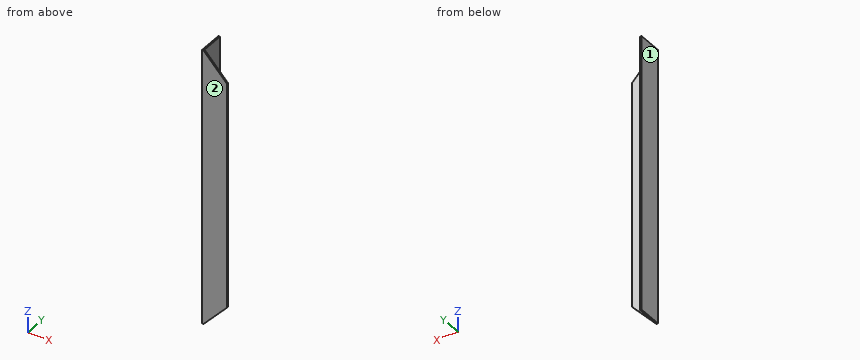
```python
from build123d import *

# Parameters (mm, degrees)
F1_DEPTH      = 533.4
F1_DEPTH_BACK = 25.4
F3_DEPTH      = 3.176


with BuildPart() as f1:
    # F0 (on Top) → F1 (new body, two sides)
    with BuildSketch(Plane.XY) as f1_sk:
        Polygon((0, 50.8), (-3.175, 50.8), (-3.175, 0), (47.625, 0), (47.625, 3.175), (0, 3.175), align=None)
    extrude(amount=F1_DEPTH)
    extrude(f1_sk.sketch, amount=-F1_DEPTH_BACK)

    # F2 (on face) → F3 (cut, through all)
    with BuildSketch(Plane(origin=(0, 3.175, 0), x_dir=(-1, 0, 0), z_dir=(0, 1, 0))):
        Polygon((-47.625, 533.4), (-47.625, 482.6), (0, 533.4), align=None)
        Polygon((0, -25.4), (-47.625, 25.4), (-47.625, -25.4), align=None)
    extrude(amount=-F3_DEPTH, mode=Mode.SUBTRACT)


solid = f1.part
```
Geometry check sheet. Reference: the model listing, model coordinates, mm. Face numbers are marked on the shaded views. Give positions to 0.01 mm unless a question says otherwise; leave off trailing zeros. Loops run counter-clockwise (first coordinate to the right, second up) from the corner with the lowest first, then second, coordinate; pieces in that order, holes last. Notation, with made-up numbers: M 31,-12 L 40,-12 A12 ccw 40,-1 Z; hole C -31.5,72.5 d11. An arc over 180 degrees is marked long. Write item = value, one per line. Start each with the question number.
1. Section check B-B, the plane x = 18. Enter the section's corners in (y, z) (3 decimals).
2. Go/stop test with flat-tipped pins: P1, Ø8, axis at y = 43, z = 92.5, coming from the +X side; P2, Ø12, axis at x = 14.5, z = 397.5, coming from the +Y side (3 decimals). Record where each tip stops, or that it passes through.
3. Section check C-C, the plane y = 17.5. Enter the section's corners in (x, z) (3 decimals).
4. Section check A-A, the plane z = 421. Enter the section's corners in (x, y) (3 decimals), plus the area to 4 significant figures.
5. Section check D-D, the plane z = 492.5. Enter the section's corners in (x, y) (3 decimals), plus the area to 3 significant figures.
6. Thickness scan on probe 1 along Y at (x, z) = (26, 364) (3 decimals); probe 2 along X at (y, z) = (34.5, 297.5) (3 decimals). Record the ranges inside material, lowest first.
7. Draft check along Y on the marked faces 1 and 2. Enter one of: +Y half, -Y half, draft (parallel to the pull), parting line (faces both ways), or undercut.
Values follow:
q1.outline = M 0,-6.2 L 3.175,-6.2 L 3.175,514.2 L 0,514.2 Z
q2.P1 = 0
q2.P2 = 3.175
q3.outline = M -3.175,-25.4 L 0,-25.4 L 0,533.4 L -3.175,533.4 Z
q4.outline = M -3.175,0 L 47.625,0 L 47.625,3.175 L 0,3.175 L 0,50.8 L -3.175,50.8 Z
q4.area = 312.5 mm^2
q5.outline = M -3.175,0 L 38.344,0 L 38.344,3.175 L 0,3.175 L 0,50.8 L -3.175,50.8 Z
q5.area = 283 mm^2
q6.probe_1 = 0 to 3.175
q6.probe_2 = -3.175 to 0
q7.face_1 = draft
q7.face_2 = -Y half
